Could you check a few things on this drawing? It's one solid part, dimensions in mm from its lowest x, y, z. Coordinates: 2 decimals unless noted, no trailing zeros. Loops run counter-clockwise (first coordinate to the right, second up) from the corner with the lowest first, then second, coordinate; pieces in that order, holes last. Notation, with made-up numbers: M 52.5,30.5 L 74.5,30.5 A23 ccw 74.5,45.5 Z; hole C 51,9.25 d1. An arc over 180 degrees is marked long. Answer as a JSON object with one key per item and string values. Group by question number.
Item 1: Suppose I cut it at C-C (z = 23). Write out the boundary of the cut face in (x, y) (1 decimal).
Item 2: Suppose I cut it at D-D (x = 41). Write out the boundary of the cut face in (y, z).
Item 3: Suppose I cut it at B-B (y = 1.1). Write out the boundary of the cut face in (x, z) (1 decimal), then the cut area to 3 significant figures.
Item 4: If I drill on line 1 (Z direction, x = 11, y = 0.5) (1 decimal); line 2 (Z direction, x = 46.5, y = 1.1) (1 decimal); line 3 (X direction, y = 0.4, z = 47) (1 decimal), over which ranges is the centre line in solid material (lowest first)?
Item 5: Suppose I cut it at A-A (z = 5.5). Write out the boundary of the cut face in (x, y) (1 decimal).
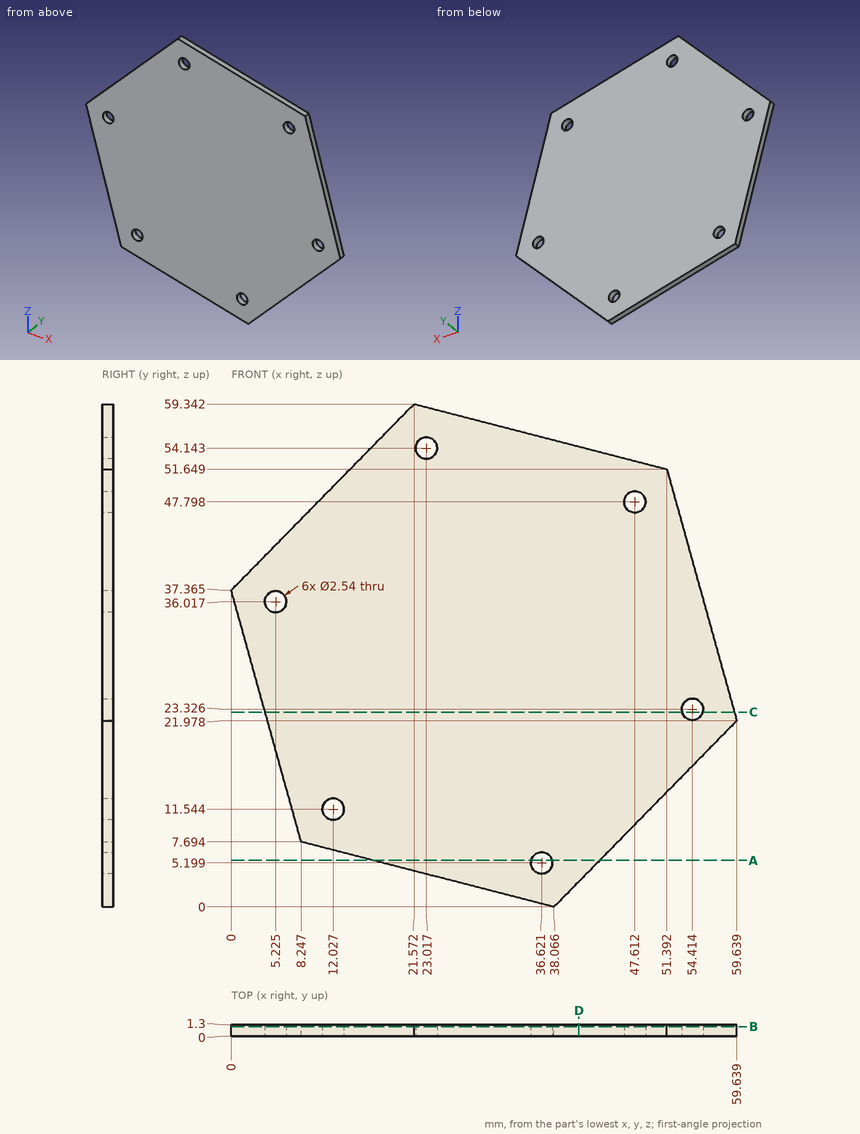
From the geometry:
{
 "1": {"outline": "M 4,0 L 53.2,0 L 53.2,1.3 L 4,1.3 Z; M 55.6,0 L 59.4,0 L 59.4,1.3 L 55.6,1.3 Z"},
 "2": {"outline": "M 0,2.99 L 1.3,2.99 L 1.3,54.33 L 0,54.33 Z"},
 "3": {"outline": "M 0,37.4 L 8.2,7.7 L 38.1,0 L 59.6,22 L 51.4,51.6 L 21.6,59.3 Z; hole C 5.2,36 d2.5; hole C 12,11.5 d2.5; hole C 23,54.1 d2.5; hole C 36.6,5.2 d2.5; hole C 47.6,47.8 d2.5; hole C 54.4,23.3 d2.5", "area": "2,430 mm2"},
 "4": {"line 1": "7 to 10.8, 12.3 to 48.6", "line 2": "8.6 to 47.2, 48.4 to 52.9", "line 3": "9.5 to 46.6, 48.6 to 52.7"},
 "5": {"outline": "M 16.7,0 L 35.4,0 L 35.4,1.3 L 16.7,1.3 Z; M 37.9,0 L 43.5,0 L 43.5,1.3 L 37.9,1.3 Z"}
}
